Design review of the part built by this model. Coordinates are the model's own, in mm. Give positions to 0.01 mm unless a question says otherwise; leave off trailing zeros. Order: outer loops, then holes, each group sorted by start corner. A loop starts at its lowest first (then second) coordinate and runs counter-clockwise, first axis right, second up.
Autodesk Inventor part; units mm, degrees
ref_plane "YZ Plane" through (0, 0, 0) normal (1, 0, 0) x (0, 1, 0)
ref_plane "XZ Plane" through (0, 0, 0) normal (0, 1, 0) x (-1, 0, 0)
ref_plane "XY Plane" through (0, 0, 0) normal (0, 0, 1) x (1, 0, 0)
sketch "Skizze1" plane through (0, 0, 0) normal (0, 0, 1) x (1, 0, 0)
  circle A0 centre (0, 0) radius 13.5
  dimension "d0" = 27
extrude "Extrusion1" add sketch "Skizze1" along normal blind 2.6
chamfer "Fase1" distance 0.5 angle 45 1 edges at (-13.5, 0, 2.6)
sketch "Skizze2" plane through (0, 0, 0) normal (0, 0, -1) x (-1, 0, 0)
  point P0 (0, 0)
  point P1 (0, 0)
hole "Bohrung1" at (0, 0, 0) direction (0, 0, 1) diameter 6.6 depth 30 tip angle 118
equation "\"d0\" = Flansch_Klemmdeckelausnahme_Dia"
equation "\"KlemmdeckelHeight\" = 3"
properties part number "Flansch_Wellennabeverbindung_Klemmdeckel" material "Edelstahl"
1. Take a section at A-A (x = 0). State the section outline as (y, z) points.
Recorded:
outline: (-13.5, 0) - (-3.3, 0) - (-3.3, 2.6) - (-13, 2.6) - (-13.5, 2.1) - close; (3.3, 0) - (13.5, 0) - (13.5, 2.1) - (13, 2.6) - (3.3, 2.6) - close
2. For line 1 along Y through (x, z) = (0, 1.6); line 2 along X through (y, z) = (2, 1.7); line 3 along Y through (x, z) = (-3, 1.5), list the stretches that pass through material, from the lowest coordinate up.
Recorded:
line 1: y = -13.5 to -3.3, 3.3 to 13.5
line 2: x = -13.35 to -2.62, 2.62 to 13.35
line 3: y = -13.16 to -1.37, 1.37 to 13.16
3. Take a section at C-C (z = 1.05). State the section outline as (x, y) points, then the cut area to 3 significant figures.
Recorded:
outline: circle Ø27 at (0, 0); hole circle Ø6.6 at (0, 0)
area: 538 mm2
4. Draft analysis for pull direction Y (two halves, no side actions). For faces 1 (the face through (3, -3, 0)), 2 (the face through (-2.23, -2.43, 1.32)), 3 (the face through (-2.93, 13.18, 1.04)), state which applies: pulls with the +Y half, pulls with the -Y half, needs draft (parallel to the pull), parting line crosses it, or undercut.
Recorded:
face 1: needs draft
face 2: undercut
face 3: parting line crosses it
5. For pin 1 (12 mm diameter, centred on x = 10.5, y = 4, fed in from -Z), flat-tipped, find the tip position at first contact; note if it passes through.
Recorded:
pin 1: stops at z = 0
